Here's how the part is built. I have some questions about the finished solid (model axes, mm). A direction names the side the tool comes from. Round coordinates to 2 decimals unless told otherwise and drop trailing zeros. Loops run counter-clockwise (first coordinate to the right, second up) from the corner with the lowest first, then second, coordinate; pieces in that order, holes last. Notation, with made-up numbers: M 7,-35.75 L 13,-35.75 A17 cw 13,-22.75 Z; hole C 71.25,-22 d10. An arc over 180 degrees is marked long. Use a Markdown table: item, result.
Autodesk Inventor part; units mm, degrees
ref_plane "YZ Plane" through (0, 0, 0) normal (1, 0, 0) x (0, 1, 0)
ref_plane "XZ Plane" through (0, 0, 0) normal (0, 1, 0) x (-1, 0, 0)
ref_plane "XY Plane" through (0, 0, 0) normal (0, 0, 1) x (1, 0, 0)
sketch "Sketch1" plane through (0, 0, 0) normal (0, 1, 0) x (-1, 0, 0)
  line L0 (22.5467, 23.3874) -> (2.5467, 23.3874)
  line L1 (2.5467, 23.3874) -> (2.5467, -6.6126)
  line L2 (2.5467, -6.6126) -> (22.5467, -6.6126)
  line L3 (22.5467, -6.6126) -> (22.5467, 23.3874)
  line L4 (12.5467, -16.022) -> (12.5467, 29.6209)
  line L5 (17.0467, 23.3874) -> (8.0467, 23.3874)
  line L6 (8.0467, 23.3874) -> (8.0467, -6.6126)
  line L7 (8.0467, -6.6126) -> (17.0467, -6.6126)
  line L8 (17.0467, -6.6126) -> (17.0467, 23.3874)
  line L9 (26.0194, 8.3874) -> (1.0659, 8.3874)
  circle A0 centre (20.0467, 13.3874) radius 1.5
  circle A1 centre (5.0467, 13.3874) radius 1.5
  circle A2 centre (20.0467, 3.3874) radius 1.5
  circle A3 centre (5.0467, 3.3874) radius 1.5
  point P0 (0, 0)
  dimension "WR" = 9
  dimension "L" = 30
  dimension "d3" = 20
  dimension "d4" = 3
  dimension "d7" = 15
  dimension "d10" = 10
extrude "Extrusion1" add sketch "Sketch1" along normal blind 8
extrude "Extrusion2" cut sketch "Sketch1" along normal blind 4 contours L8 L9 L4 L0 | L4 L9 L6 L0 | L8 L2 L4 L9 | L4 L2 L6 L9
properties part number "slider-slider"
Q1. Imagine slicing it at A-A, the plane y = 2.25. Please give me the cut outline in (x, z).
Return value:
| item | result |
|---|---|
| outline | M -22.55,-6.61 L -17.05,-6.61 L -17.05,23.39 L -22.55,23.39 Z; M -8.05,-6.61 L -2.55,-6.61 L -2.55,23.39 L -8.05,23.39 Z; hole C -20.05,3.39 d3; hole C -20.05,13.39 d3; hole C -5.05,3.39 d3; hole C -5.05,13.39 d3 |
Q2. I need wall thicknesses on line 1 (Z direction, x = -5.5, y = 2.5); line 2 (X direction, y = 3, z = -2.5); line 3 (Z direction, x = -6.25, y = 7.75). Which ranges of each line are inside material? Lowest first, please. Write a range as from..to.
Return value:
| item | result |
|---|---|
| line 1 | z = -6.61..1.96, 4.82..11.96, 14.82..23.39 |
| line 2 | x = -22.55..-17.05, -8.05..-2.55 |
| line 3 | z = -6.61..2.49, 4.28..12.49, 14.28..23.39 |
Q3. Will these pins go through, and if not, where does the flat tip stop? P1, Ø1, axis at x = -16, y = 1.5, coming from the +Z side; P2, Ø4.5, axis at x = -13.5, z = 9.5, coming from the -Y side.
Return value:
| item | result |
|---|---|
| P1 | passes through |
| P2 | stops at y = 4 |
Q4. Imagine slicing it at C-C, the plane y = 7. Please give me the cut outline in (x, z), then the cut area to 3 significant figures.
Return value:
| item | result |
|---|---|
| outline | M -22.55,-6.61 L -2.55,-6.61 L -2.55,23.39 L -22.55,23.39 Z; hole C -20.05,3.39 d3; hole C -20.05,13.39 d3; hole C -5.05,3.39 d3; hole C -5.05,13.39 d3 |
| area | 572 mm^2 |
Q5. Imagine slicing it at B-B, the plane z = 3.75. Please give me the cut outline in (x, y).
Return value:
| item | result |
|---|---|
| outline | M -22.55,0 L -21.5,0 L -21.5,8 L -22.55,8 Z; M -18.59,0 L -17.05,0 L -17.05,4 L -8.05,4 L -8.05,0 L -6.5,0 L -6.5,8 L -18.59,8 Z; M -3.59,0 L -2.55,0 L -2.55,8 L -3.59,8 Z |
Q6. We'd pull the mould along X, two halves only. Please class faces 3 (the flat face through (-5, 0, 9)), 4 (the cylindrical face through (-3.941, 3.944, 12.374)), 5 (the flat face through (-22.547, 4, 8)): pulls with the +X half, pulls with the -X half, needs draft (parallel to the pull), parting line crosses it, or undercut.
Return value:
| item | result |
|---|---|
| face 3 | needs draft |
| face 4 | undercut |
| face 5 | pulls with the -X half |
Q7. Imagine slicing it at D-D, the plane z = 16.5. Please give me the cut outline in (x, y).
Return value:
| item | result |
|---|---|
| outline | M -22.55,0 L -17.05,0 L -17.05,4 L -8.05,4 L -8.05,0 L -2.55,0 L -2.55,8 L -22.55,8 Z |
Q8. For faces 1 (the flat face through (-8.047, 2, 9)), 2 (the flat face through (-2.547, 4, 9)), which set-ups out of +Z, -Z, +X, -X, +Y, -Y let a thin tool reach every point of the face, with its end or its side?
Return value:
| item | result |
|---|---|
| face 1 | +Z, -Z, -Y |
| face 2 | +Z, -Z, +X, +Y, -Y |
